from build123d import *

# Parameters (mm, degrees)
F0_R     = 11.65
F0_R_2   = 11
F1_DEPTH = 220
F3_DEPTH = 0.8
F4_COUNT = 5


with BuildPart() as f1:
    # F0 (on Front) → F1 (new body)
    with BuildSketch(Plane.XZ):
        Circle(F0_R)
        Circle(F0_R_2, mode=Mode.SUBTRACT)
    extrude(amount=F1_DEPTH)

    # F2 (on Right) → F3 (join)
    with BuildSketch(Plane.YZ):
        Polygon((-60.803428, 10.931599), (0, 10.931599), (0, 24.654245), (-30.401714, 18.606978), (-41.75102, 18.382577), align=None)
    extrude(amount=F3_DEPTH)

    # F4: F1 ×5 about axis
    f4_axis = Axis((0, 0, 0), (0, -1, 0))


with BuildPart() as f1_1:
    add(f1.part)
    for i in range(1, F4_COUNT):
        add(f1.part.rotate(f4_axis, i * 360 / F4_COUNT))


solid = f1_1.part
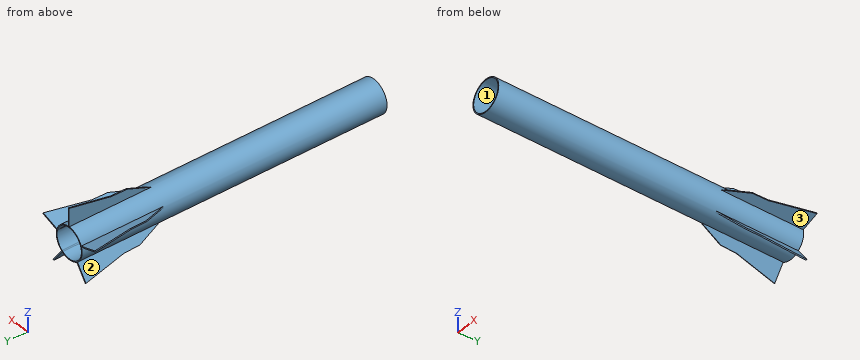
Could you check a few things on this model? Use its own coordinates, in mm. Face numbers are marked on the shaded views. Give positions to 0.01 mm unless a question says otherwise; leave off trailing zeros. Write each loop counter-clockwise with the first axis right and the second up, starting at its lowest first coordinate (ties: lowest second). Pieces come first, ordered by that corner, then holes. Notation, with made-up numbers: (-25, -32) - (18, -32) arc R20 ccw to (18, -23) - close; hole circle Ø5 at (-9.5, 12.5). An arc over 180 degrees is marked (long way). Use CSV: the item, a comma, the result in double quotes. Start each with the question number.
Item 1: I want a section at A-A, the plane z = 0. Please give me the cut outline in (x, y), then the cut area to 3 significant figures.
Item 2: I'm going to push flat-ended pins straight in: pin 1 (3 mm diameter, centred on y = -61.5, z = 4, fed in from -X); pin 2 (2 mm diameter, centred on x = -7.5, y = -147, fed in from +Z); pin 3 (3 mm diameter, centred on y = -46, z = -12, fed in from -X). Where does each tip first touch, or does it pass through?
Item 3: I want a section at C-C, the plane y = -136. Please give me the cut outline in (x, z).
Item 4: If we mould it in two halves opening along X, with no side actions, what happens to the marked faces 1, 2 and 3? For each: pulls with the +X half, pulls with the -X half, needs draft (parallel to the pull), parting line crosses it, or undercut.
Item 5: I want a section at D-D, the plane z = 20.5. Please give me the cut outline in (x, y), then the cut area to 3 significant figures.
Item 6: If I drill on line 1 along Z through (x, y) = (0, -112.5); line 2 along Z through (x, y) = (8, -105.5), over which ranges is the centre line in solid material (lowest first)?
Item 7: I want a section at B-B, the plane x = 3. Please give me the cut outline in (y, z), then the cut area to 3 significant figures.
Findings:
1,outline,"(-11.65, -220) - (-11, -220) - (-11, 0) - (-11.65, 0) - close; (11, -220) - (11.65, -220) - (11.65, 0) - (11, 0) - close"
1,area,"286 mm2"
2,pin 1,"stops at x = -11.38"
2,pin 2,"stops at z = 9.67"
2,pin 3,"stops at x = -10.65"
3,outline,"circle Ø23.3 at (0, 0); hole circle Ø22 at (0, 0)"
4,face 1,"undercut"
4,face 2,"pulls with the -X half"
4,face 3,"pulls with the +X half"
5,outline,"(0, -20.88) - (0.8, -20.88) - (0.8, 0) - (0, 0) - close"
5,area,"16.7 mm2"
6,line 1,"z = -11.65 to -11, 11 to 11.65"
6,line 2,"z = -8.47 to -7.55, 7.55 to 8.47"
7,outline,"(-220, -11.26) - (0, -11.26) - (0, -10.58) - (-220, -10.58) - close; (-220, 10.58) - (0, 10.58) - (0, 11.26) - (-220, 11.26) - close"
7,area,"297 mm2"
